CAD build for the part. Positions are in the model's coordinates, mm. Face numbers are marked on the shaded views. Give positions to 0.01 mm unless a question says otherwise; leave off trailing zeros. Order: outer loops, then holes, each group sorted by start corner. A loop starts at its lowest first (then second) coordinate and runs counter-clockwise, first axis right, second up.
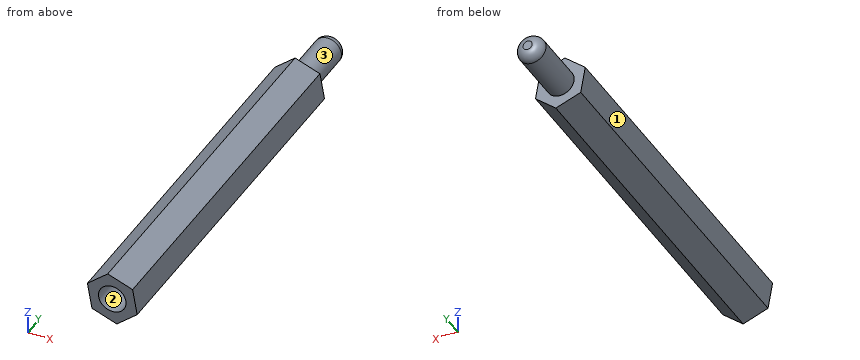
```python
from build123d import *

# Parameters (mm, degrees)
BOSS_EXTRUDE1_DEPTH = 40
SKETCH2_R           = 1.5
BOSS_EXTRUDE2_DEPTH = 7
SKETCH3_R           = 1.5
CUT_EXTRUDE1_DEPTH  = 7
FILLET1_R           = 1


with BuildPart() as part:
    # Sketch1 → Boss-Extrude1 (new body)
    with BuildSketch(Plane(origin=(0, 0, 0), x_dir=(1, 0, 0), z_dir=(0, 1, 0))):
        Polygon((2.214824591, -1.851454932), (2.7108193, 0.992366895), (0.495994709, 2.843821827), (-2.214824591, 1.851454932), (-2.7108193, -0.992366895), (-0.495994709, -2.843821827), align=None)
    extrude(amount=BOSS_EXTRUDE1_DEPTH)

    # Sketch2 → Boss-Extrude2 (add)
    with BuildSketch(Plane(origin=(0, 40, 0), x_dir=(1, 0, 0), z_dir=(0, 1, 0))):
        Circle(SKETCH2_R)
    extrude(amount=BOSS_EXTRUDE2_DEPTH)

    # Sketch3 → Cut-Extrude1 (cut)
    with BuildSketch(Plane.XZ):
        Circle(SKETCH3_R)
    extrude(amount=-CUT_EXTRUDE1_DEPTH, mode=Mode.SUBTRACT)

    # Fillet1
    fillet1_edges = [part.edges().sort_by_distance(p)[0] for p in [
        (-1.5, 47, 0),
    ]]
    fillet(fillet1_edges, radius=FILLET1_R)


solid = part.part
```
Item 1: Two-plate mould, pull along Z, no slides. Class the marked faces 1, 2 and 3: released by +Z, released by -Z, zero draft, split by the parting line, or undercut.
Item 2: Slice it at A-A (y = 38.5). Give the cut face in (x, z), and give its area (3 significant figures).
Item 3: Slice it at B-B (z = -2.25). Give the cut face in (x, y), and give its area (3 significant figures).
Item 4: Drop flat-ended pins along their axis: pin 1 Ø1 at (x, z) = (1.5, -0.5) entering from +Y; pin 2 Ø1 at (y, z) = (37, 0) entering from +X; pin 3 Ø2 at (y, z) = (38, -1.5) entering from -X. Give the stop position or say it passes through.
Item 5: Wall check: L1, parallel to Y at x = -1.75, z = -0.95; L2, parallel to Z at x = 0, y = 5; L3, parallel to X at y = 4, z = 0.6. Give the ranges that are in metal, low to high.
A:
1. face 1: released by -Z
1. face 2: undercut
1. face 3: split by the parting line
2. outline: (-2.71, 0.99) - (-2.21, -1.85) - (0.5, -2.84) - (2.71, -0.99) - (2.21, 1.85) - (-0.5, 2.84) - close
2. area: 21.7 mm2
3. outline: (-1.13, 0) - (1.21, 0) - (1.21, 40) - (-1.13, 40) - close
3. area: 93.3 mm2
4. pin 1: stops at y = 46.81
4. pin 2: stops at x = 2.62
4. pin 3: stops at x = -2.45
5. L1: y = 0 to 40
5. L2: z = -2.66 to -1.5, 1.5 to 2.66
5. L3: x = -2.64 to -1.37, 1.37 to 2.43
